Can you work these out from the model? Positions are in its coordinate system, mm. Face numbers are marked on the shaded views. A direction names the side the tool comes from. Give positions to 0.01 mm unless a question says otherwise; leave off trailing zeros. Loops run counter-clockwise (first coordinate to the right, second up) from the corner with the lowest first, then second, coordinate; pieces in that order, holes last. Notation, with made-up numbers: M 11,-37.5 L 23,-37.5 A6 ccw 23,-31.5 Z; hole C 46,51 d1. An arc over 180 degrees is marked long. Put each result on its own line as item: value. Start each with the question number.
1) For the marked faces 5 and 6, which set-ups out of +Z, -Z, +X, -X, +Y, -Y let a thin tool reach every point of the face, with its end or its side?
2) Imagine slicing it at A-A (x = 0). Write out the boundary of the cut face in (y, z) (3 decimals), then the cut area to 3 significant figures.
3) If we mould it in two halves opening along X, with no side actions, what happens to the marked faces 1, 2, 3 and 4? For each: +X half, -X half, draft (parallel to the pull), parting line (faces both ways), or undercut.
4) Imagine slicing it at C-C (z = 0). State how many separate pieces and enclosed holes the cut face has, then the cut area to 3 significant figures.
5) Please list where these lines run through material, in increasing order: line 1 along X through (y, z) = (3.25, 1.5); line 2 along X through (y, z) = (3.75, -5.25); line 3 along Z through (x, y) = (0, 2.75). Write a range as from..to.
6) For P1, Ø2, axis at x = 17, y = 4, coming from the +Z side; P2, Ø5, axis at x = -6.5, y = 5.5, coming from the -Z side; P3, Ø0.6, axis at x = -11, z = 0, coming from the -Y side, each with a flat end and sliding along its axis, tell me the tip position at first contact or that it passes through.
7) Imagine slicing it at B-B (y = 1). Write out the boundary of the cut face in (x, z).
8) Imagine slicing it at D-D (x = 18.25). Write out the boundary of the cut face in (y, z).
from build123d import *

# Parameters (mm, degrees)
SKETCH1_R              = 11
FLANGE_DEPTH           = 4
SKETCH3_R              = 13.425
TOP_RECESS_DEPTH       = 0.5
BOTTOM_RECESS_1_DEPTH  = 0.5
BOTTOM_RECESS_2_DEPTH  = 3
MOUNTING_HOLE_M5X0_8_D = 5


with BuildPart() as part:
    # Sketch1 → Flange (new body)
    with BuildSketch(Plane(origin=(0, 0, 0), x_dir=(1, 0, 0), z_dir=(0, 1, 0))):
        with BuildLine():
            Line((20.578767123, 4.424572712), (6.287671233, 11.946346323))
            ThreePointArc((6.287671233, 11.946346323), (0, 13.5), (-6.287671233, 11.946346323))
            Line((-6.287671233, 11.946346323), (-20.578767123, 4.424572712))
            ThreePointArc((-20.578767123, 4.424572712), (-23.25, 0), (-20.578767123, -4.424572712))
            Line((-20.578767123, -4.424572712), (-6.287671233, -11.946346323))
            ThreePointArc((-6.287671233, -11.946346323), (0, -13.5), (6.287671233, -11.946346323))
            Line((6.287671233, -11.946346323), (20.578767123, -4.424572712))
            ThreePointArc((20.578767123, -4.424572712), (23.25, 0), (20.578767123, 4.424572712))
        make_face()
        with Locations(Location((0, 0, 0), (0, 0, 270))):
            Circle(SKETCH1_R, mode=Mode.SUBTRACT)
    extrude(amount=FLANGE_DEPTH)

    # Sketch2 → Bearing Seat (revolve)
    with BuildSketch(Plane.XY, mode=Mode.PRIVATE) as bearing_seat_sk:
        Polygon((-13.425, 4), (-12.675, 8.5), (-11.3, 8.5), (-11.3, 8), (-11, 8), (-11, 4), align=None)
    revolve(bearing_seat_sk.sketch.rotate(Axis((0, 0, 0), (0, 1, 0)), 270), axis=Axis((0, 0, 0), (0, 1, 0)))

    # Sketch3 → Top Recess (cut)
    with BuildSketch(Plane(origin=(0, 4, 0), x_dir=(1, 0, 0), z_dir=(0, 1, 0))):
        with BuildLine():
            Line((10.970198855, 9.481810855), (6.287671233, 11.946346323))
            ThreePointArc((6.287671233, 11.946346323), (0, 13.5), (-6.287671233, 11.946346323))
            Line((-6.287671233, 11.946346323), (-10.970198855, 9.481810855))
            ThreePointArc((-10.970198855, 9.481810855), (-14.5, 0), (-10.970198855, -9.481810855))
            Line((-10.970198855, -9.481810855), (-6.287671233, -11.946346323))
            ThreePointArc((-6.287671233, -11.946346323), (0, -13.5), (6.287671233, -11.946346323))
            Line((6.287671233, -11.946346323), (10.970198855, -9.481810855))
            ThreePointArc((10.970198855, -9.481810855), (14.5, 0), (10.970198855, 9.481810855))
        make_face()
        with Locations(Location((0, 0, 0), (0, 0, 270))):
            Circle(SKETCH3_R, mode=Mode.SUBTRACT)
    extrude(amount=-TOP_RECESS_DEPTH, mode=Mode.SUBTRACT)

    # Sketch5 → Bottom Recess 1 (cut)
    with BuildSketch(Plane.XZ):
        with BuildLine():
            Line((17.009424329, 4.325618107), (5.47260274, 10.397745874))
            ThreePointArc((5.47260274, 10.397745874), (0, 11.75), (-5.47260274, 10.397745874))
            Line((-5.47260274, 10.397745874), (-17.009424329, 4.325618107))
            ThreePointArc((-17.009424329, 4.325618107), (-13.75, 0), (-17.009424329, -4.325618107))
            Line((-17.009424329, -4.325618107), (-5.47260274, -10.397745874))
            ThreePointArc((-5.47260274, -10.397745874), (0, -11.75), (5.47260274, -10.397745874))
            Line((5.47260274, -10.397745874), (17.009424329, -4.325618107))
            ThreePointArc((17.009424329, -4.325618107), (13.75, 0), (17.009424329, 4.325618107))
        make_face()
    extrude(amount=-BOTTOM_RECESS_1_DEPTH, mode=Mode.SUBTRACT)

    # Sketch6 → Bottom Recess 2 (cut)
    with BuildSketch(Plane.XZ.offset(-0.5)):
        with BuildLine():
            Line((-11.01986842, 4.75), (11.01986842, 4.75))
            ThreePointArc((11.01986842, 4.75), (12, 0), (11.01986842, -4.75))
            Line((11.01986842, -4.75), (-11.01986842, -4.75))
            ThreePointArc((-11.01986842, -4.75), (-12, 0), (-11.01986842, 4.75))
        make_face()
    extrude(amount=-BOTTOM_RECESS_2_DEPTH, mode=Mode.SUBTRACT)

    # Mounting Hole (M5x0.8) (through all)
    with Locations(Plane(origin=(0, 4, 0), x_dir=(1, 0, 0), z_dir=(0, 1, 0))):
        with Locations((18.25, 0), (-18.25, 0)):
            Hole(MOUNTING_HOLE_M5X0_8_D / 2)


solid = part.part
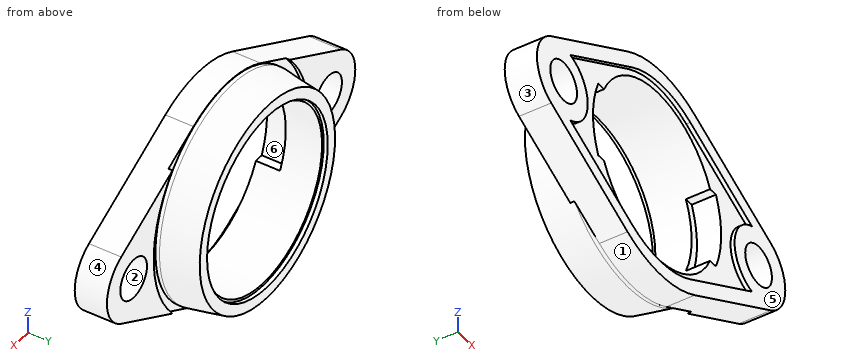
Recorded:
1. face 5: +Z, -Z, +X, -X, -Y
1. face 6: -Y
2. outline: M 0,-13.5 L 3.5,-13.5 L 3.5,-13.425 L 4,-13.425 L 8.5,-12.675 L 8.5,-11.3 L 8,-11.3 L 8,-11 L 0.5,-11 L 0.5,-11.75 L 0,-11.75 Z; M 0,11.75 L 0.5,11.75 L 0.5,11 L 8,11 L 8,11.3 L 8.5,11.3 L 8.5,12.675 L 4,13.425 L 3.5,13.425 L 3.5,13.5 L 0,13.5 Z
2. area: 37.3 mm²
3. face 1: parting line
3. face 2: undercut
3. face 3: -X half
3. face 4: +X half
4. separate pieces: 4
4. enclosed holes: 0
4. area: 66.3 mm²
5. line 1: -23.02..-20.25, -16.25..-11.91, 11.91..16.25, 20.25..23.02
5. line 2: -19.01..-13.52, -12.36..-9.67, 9.67..12.36, 13.52..19.01
5. line 3: -13.5..-11, 11..13.5
6. P1: z = 6.83
6. P2: z = -12.66
6. P3: y = 3.5
7. outline: M -20.58,-4.42 L -6.29,-11.95 A13.5 ccw 6.29,-11.95 L 20.58,-4.42 A5 ccw 20.58,4.42 L 6.29,11.95 A13.5 ccw -6.29,11.95 L -20.58,4.42 A5 ccw Z; hole C -18.25,0 d5; hole M -11.02,-4.75 L -9.92,-4.75 A11 ccw 9.92,-4.75 L 11.02,-4.75 A12 ccw 11.02,4.75 L 9.92,4.75 A11 ccw -9.92,4.75 L -11.02,4.75 A12 ccw Z; hole C 18.25,0 d5
8. outline: M 0,-5.65 L 4,-5.65 L 4,-2.5 L 0,-2.5 Z; M 0,2.5 L 4,2.5 L 4,5.65 L 0,5.65 Z
